Design review of the part built by this model. Coordinates are the model's own, in mm. Face numbers are marked on the shaded views. Round coordinates to 2 decimals unless told otherwise and drop trailing zeros. Loops run counter-clockwise (first coordinate to the right, second up) from the corner with the lowest first, then second, coordinate; pieces in that order, holes last. Notation, with made-up numbers: (-14.75, 66.25) - (19.25, 66.25) arc R23 ccw to (19.25, 98.25) - close; hole circle Ø6 at (-12.75, 84.5). An arc over 180 degrees is marked (long way). Answer as CSV lines item,"result". Start each with the question number.
(1) Mouldability with a two-part tool opening along Y and no side actions: class the marked faces 1, 2 and 3 as released by +Y, released by -Y, zero draft, split by the parting line, or undercut.
(2) Consider section B-B (y = 27.5). Give the boundary of the cut face in (x, z), and give its area (3 significant figures).
(3) Consider section C-C (x = 82.5). Give the boundary of the cut face in (y, z), and give its area (3 significant figures).
(4) Consider section D-D (z = 91). Give the boundary of the cut face in (x, y).
(5) Wall thickness on L1, parallel to X at y = 3, z = 44; L2, parallel to X at y = 27, z = 44.87: over which ranges is each line inside the solid? List them lowest first.
(6) Consider section A-A (y = 17). Give the boundary of the cut face in (x, z), and give its area (3 significant figures).
(7) For P1, Ø1.2, axis at x = 83, z = 44.5, coming from the -Y side; P2, Ø3, axis at y = 9, z = 39, coming from the +X side; P3, Ø1.2, axis at x = 82.5, z = 45.5, coming from the +Y side, all flat-tipped, find the tip position at first contact; note any pin that passes through.
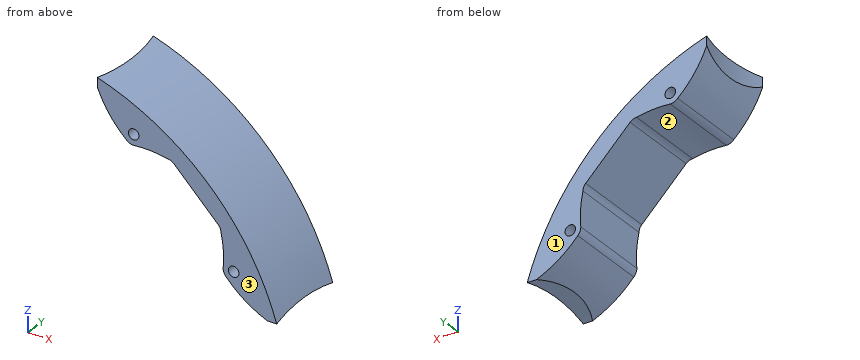
Autodesk Inventor part; units mm, degrees
ref_plane "YZ Plane" through (0, 0, 0) normal (1, 0, 0) x (0, 1, 0)
ref_plane "XZ Plane" through (0, 0, 0) normal (0, 1, 0) x (-1, 0, 0)
ref_plane "XY Plane" through (0, 0, 0) normal (0, 0, 1) x (1, 0, 0)
sketch "Эскиз1" plane through (0, 0, 0) normal (0, 1, 0) x (-1, 0, 0)
  arc A0 (-31, 99.2724) -> (-99.2724, 31) centre (0, 0) ccw
  circle A1 centre (-74.5664, 57.67) radius 1.5
  circle A2 centre (-82.9015, 44.87) radius 1.5
  circle A3 centre (-57.67, 74.5664) radius 1.5
  circle A4 centre (-44.87, 82.9015) radius 1.5
  line L0 (-31, 99.2724) -> (-31, 78.7724)
  line L1 (-31, 78.7724) -> (31, 78.7724)
  circle A5 centre (-16, 72.43) radius 1.5
  circle A6 centre (16, 72.43) radius 1.5
  circle A7 centre (31, 72.43) radius 1.5
  line L2 (31, 78.7724) -> (31, 99.2724)
  circle A8 centre (16, 42.22) radius 1.5
  circle A9 centre (-16, 42.22) radius 1.5
  circle A10 centre (-42.22, 16) radius 1.5
  circle A11 centre (-72.43, 16) radius 1.5
  line L3 (-99.2724, 31) -> (-78.7724, 31)
  line L4 (-78.7724, 31) -> (-78.7724, -31)
  arc A12 (34.57, 98.0863) -> (98.0863, 34.57) centre (109.0212, 109.0212) ccw
  circle A13 centre (72.43, 31) radius 1.5
  line L5 (99.2724, 31) -> (78.7724, 31)
  line L6 (78.7724, 31) -> (78.7724, -31)
  circle A14 centre (72.43, 16) radius 1.5
  circle A15 centre (42.22, 16) radius 1.5
  circle A16 centre (42.22, -16) radius 1.5
  circle A17 centre (72.43, -16) radius 1.5
  circle A18 centre (82.9015, -44.87) radius 1.5
  line L7 (78.7724, -31) -> (99.2724, -31)
  arc A19 (31, -99.2724) -> (99.2724, -31) centre (0, 0) ccw
  circle A20 centre (74.5664, -57.67) radius 1.5
  circle A21 centre (16, -42.22) radius 1.5
  circle A22 centre (57.67, -74.5664) radius 1.5
  circle A23 centre (44.87, -82.9015) radius 1.5
  circle A24 centre (16, -72.43) radius 1.5
  line L8 (31, -78.7724) -> (31, -99.2724)
  line L9 (-31, -78.7724) -> (31, -78.7724)
  circle A25 centre (-16, -72.43) radius 1.5
  circle A26 centre (-16, -42.22) radius 1.5
  circle A27 centre (-31, -72.43) radius 1.5
  circle A28 centre (-42.22, -16) radius 1.5
  circle A29 centre (-72.43, -16) radius 1.5
  circle A30 centre (-72.43, -31) radius 1.5
  line L10 (-78.7724, -31) -> (-99.2724, -31)
  line L11 (-31, -99.2724) -> (-31, -78.7724)
  arc A31 (-34.57, -98.0863) -> (-31, -99.2724) centre (0, 0) ccw
  arc A32 (-99.2724, -31) -> (-98.0863, -34.57) centre (0, 0) ccw
  arc A33 (-34.57, -98.0863) -> (-98.0863, -34.57) centre (-109.0212, -109.0212) ccw
  line L12 (-73.5391, 73.5391) -> (73.5391, -73.5391) construction
  arc A34 (34.57, 98.0863) -> (31, 99.2724) centre (0, 0) ccw
  arc A35 (99.2724, 31) -> (98.0863, 34.57) centre (0, 0) ccw
  arc A36 (-98.0863, -34.57) -> (-34.57, -98.0863) centre (0, 0) ccw
  arc A37 (98.0863, 34.57) -> (34.57, 98.0863) centre (0, 0) ccw
sketch "Эскиз2" plane through (0, 0, 0) normal (0, 1, 0) x (-1, 0, 0)
  circle A0 centre (-82.9015, 44.87) radius 1.5
  circle A1 centre (-44.87, 82.9015) radius 1.5
  circle A2 centre (-44.87, 82.9015) radius 2
  circle A3 centre (-82.9015, 44.87) radius 2
  arc A4 (-31, 99.2724) -> (-99.2724, 31) centre (0, 0) ccw
  arc A5 (-31, 99.2724) -> (-99.2724, 31) centre (0, 0) ccw
  circle A6 centre (-44.87, 82.9015) radius 4
  circle A7 centre (-82.9015, 44.87) radius 4
  line L0 (-73.5391, 73.5391) -> (73.5391, -73.5391) construction
  line L1 (-31, 99.2724) -> (-31, 78.7724)
  line L2 (-99.2724, 31) -> (-78.7724, 31)
  arc A8 (-31, 95.7724) -> (-95.7724, 31) centre (0, 0) ccw construction
  line L3 (-31, 95.7724) -> (-95.7724, 31) construction
  line L4 (-42.0416, 85.7299) -> (-47.6984, 80.0731) construction
  circle A9 centre (-57.67, 74.5664) radius 1.5 construction
  circle A10 centre (-74.5664, 57.67) radius 1.5 construction
  circle A11 centre (-57.67, 74.5664) radius 3.5
  circle A12 centre (-74.5664, 57.67) radius 3.5
  line L5 (-60.1449, 77.0413) -> (-55.1951, 72.0915) construction
  line L6 (-77.0413, 60.1449) -> (-72.0915, 55.1951) construction
  line L7 (-60.1449, 77.0413) -> (-77.0413, 60.1449)
  line L8 (-44.87, 82.9015) -> (-42.0416, 80.0731) construction
  arc A13 (-42.0416, 80.0731) -> (-31, 95.7724) centre (-70.386, 111.7408) ccw
  line L9 (-42.0416, 80.0731) -> (-47.6984, 80.0731) construction
  line L10 (-44.87, 82.9015) -> (-44.87, 78.9015) construction
  line L11 (-55.1951, 77.0413) -> (-60.1449, 72.0915) construction
  line L12 (-60.1449, 77.0413) -> (-55.1951, 77.0413) construction
  line L13 (-57.67, 74.5664) -> (-57.67, 78.0664) construction
  arc A14 (-44.87, 78.9015) -> (-57.67, 78.0664) centre (-48.6366, 38.1205) ccw
  arc A15 (-78.0664, 57.67) -> (-78.9015, 44.87) centre (-38.1205, 48.6366) ccw
  line L14 (-82.9015, 44.87) -> (-80.0731, 42.0416) construction
  arc A16 (-95.7724, 31) -> (-80.0731, 42.0416) centre (-111.7408, 70.386) ccw
  point P0 (-95.7724, 31)
  point P1 (-95.7724, 31)
  point P2 (-78.9015, 44.87)
  dimension "d3" = 8
  dimension "d0" = 4
  dimension "d1" = 4
  dimension "d2" = 8
  dimension "d4" = 3.5
  dimension "d5" = 3.5
  dimension "d7" = 7
  dimension "d8" = 7
  dimension "d9" = 42.5
extrude "Выдавливание1" add sketch "Эскиз2" along normal blind 32 contours L1 A13 A6 A14 A11 L7 A12 A15 A7 A16 L2 A4 | A6 A14 | A7 A15 picked at (-41.5746, 83.2174) picked at (-80.8909, 42.2371)
ref_plane "РабПлоскость1" through (0, 25.3, 0) normal (0, 1, 0) x (1, 0, 0)
sketch "Эскиз3" plane through (0, 25.3, 0) normal (0, 1, 0) x (1, 0, 0)
  circle A0 centre (44.87, -82.9015) radius 2
  circle A1 centre (82.9015, -44.87) radius 2
  point P0 (0, 0)
extrude "Выдавливание2" add sketch "Эскиз3" against normal blind 20.6
ref_plane "РабПлоскость2" through (99.2724, 32, 31) normal (1, 0, 0) x (0, -1, 0)
sketch "Эскиз4" plane through (99.2724, 32, 31) normal (1, 0, 0) x (0, -1, 0)
  arc A0 (0, 0) -> (32, 0) centre (16, 72.5568) ccw
  line L0 (32, 0) -> (0, 0)
  line L1 (0, 0) -> (32, 0)
  point P0 (32, 31)
  dimension "d15" = 74.3
extrude "Выдавливание3" cut sketch "Эскиз4" against normal blind 20.6
ref_plane "РабПлоскость3" through (73.5391, 32, 73.5391) normal (0.7071, 0, -0.7071) x (0, -1, 0)
mirror "Зеркальное отражение1" about plane through (73.5391, 32, 73.5391) normal (0.7071, 0, -0.7071) of "Выдавливание3"
properties part number "protect"
Determined:
1,face 1,"released by +Y"
1,face 2,"zero draft"
1,face 3,"released by -Y"
2,outline,"(31.85, 93.82) arc R42.5 ccw to (42.04, 80.07) arc R4 ccw to (44.87, 78.9) arc R40.95 cw to (57.67, 78.07) arc R3.5 cw to (60.14, 77.04) - (77.04, 60.14) arc R3.5 cw to (78.07, 57.67) arc R40.95 cw to (78.9, 44.87) arc R4 ccw to (80.07, 42.04) arc R42.5 ccw to (93.82, 31.85) - (99, 31.85) arc R104 ccw to (31.85, 99) - close; hole circle Ø4 at (44.87, 82.9); hole circle Ø4 at (82.9, 44.87)"
2,area,"821 mm^2"
3,outline,"(0, 39.54) - (32, 39.54) - (32, 42.91) - (25.3, 42.91) - (25.3, 46.83) - (32, 46.83) - (32, 63.32) - (0, 63.32) - (0, 46.83) - (4.7, 46.83) - (4.7, 42.91) - (0, 42.91) - close"
3,area,"716 mm^2"
4,outline,"(33.29, 0) - (50.35, 0) - (50.35, 32) - (33.29, 32) - close"
5,L1,"x = 79 to 81.1, 84.7 to 94.23"
5,L2,"x = 78.9 to 80.9, 84.9 to 93.82"
6,outline,"(32.74, 92.02) arc R42.5 ccw to (42.04, 80.07) arc R4 ccw to (44.87, 78.9) arc R40.95 cw to (57.67, 78.07) arc R3.5 cw to (60.14, 77.04) - (77.04, 60.14) arc R3.5 cw to (78.07, 57.67) arc R40.95 cw to (78.9, 44.87) arc R4 ccw to (80.07, 42.04) arc R42.5 ccw to (92.02, 32.74) - (98.71, 32.74) arc R104 ccw to (32.74, 98.71) - close"
6,area,"836 mm^2"
7,P1,"stops at y = 4.7"
7,P2,"stops at x = 97"
7,P3,"stops at y = 25.3"
